Read the model definition and answer for the solid it produces. Units are mm, in the model's axes. A direction names the side the tool comes from. Round coordinates to 2 decimals unless told otherwise and drop trailing zeros. Write each loop counter-clockwise with the first axis right and the second up, starting at its lowest first coordinate (ties: lowest second). Pieces come first, ordered by that corner, then holes. Notation, with made-up numbers: (49, -23) -> (84, -23) arc R27 cw to (84, 0) -> close; hole circle Ø5 at (48, 16.5). An arc over 180 degrees is marked (long way). Return JSON: item names as keys, results as strings.
from build123d import *

# Parameters (mm, degrees)
F0_W     = 27
F0_H     = 19
F1_DEPTH = 2
F2_R     = 3.5
F3_R     = 0.5


with BuildPart() as f1:
    # F0 (on Front) → F1 (new body)
    with BuildSketch(Plane.XZ):
        with Locations((-46.395146, 6.552132)):
            Rectangle(F0_W, F0_H)
        with BuildLine():
            ThreePointArc((-45.395146, 12.252132), (-43.895146, 13.752132), (-42.395146, 12.252132))
            Line((-42.395146, 12.252132), (-42.395146, 8.716104))
            Line((-42.395146, 8.716104), (-39.834486, 6.155444))
            ThreePointArc((-39.834486, 6.155444), (-39.509326, 5.668809), (-39.395146, 5.094783))
            Line((-39.395146, 5.094783), (-39.395146, 2.152132))
            ThreePointArc((-39.395146, 2.152132), (-39.834486, 1.091472), (-40.895146, 0.652132))
            Line((-40.895146, 0.652132), (-43.895146, 0.652132))
            ThreePointArc((-43.895146, 0.652132), (-44.955806, 1.091472), (-45.395146, 2.152132))
            Line((-45.395146, 2.152132), (-45.395146, 2.652132))
            ThreePointArc((-45.395146, 2.652132), (-44.908531, 3.758048), (-43.764412, 4.146424))
            Line((-43.764412, 4.146424), (-41.90547, 3.983787))
            Line((-41.90547, 3.983787), (-41.955806, 4.034123))
            Line((-41.955806, 4.034123), (-45.395146, 7.473463))
            Line((-45.395146, 7.473463), (-45.395146, 12.252132))
        make_face(mode=Mode.SUBTRACT)
    extrude(amount=F1_DEPTH)

    # F2
    f2_edges = [f1.edges().sort_by_distance(p)[0] for p in [
        (-45.395146, -1, 7.473463),
    ]]
    fillet(f2_edges, radius=F2_R)

    # F3
    f3_edges = [f1.edges().sort_by_distance(p)[0] for p in [
        (-42.395146, -1, 8.716104),
    ]]
    fillet(f3_edges, radius=F3_R)


solid = f1.part
Item 1: Section B-B (y = -0.65) is taken. Give the vertices of the cut face in (x, z), then the cut area to 3 significant figures.
Worked answers:
{"outline": "(-59.9, -2.95) -> (-32.9, -2.95) -> (-32.9, 16.05) -> (-59.9, 16.05) -> close; hole (-45.4, 2.15) arc R1.5 ccw to (-43.9, 0.65) -> (-40.9, 0.65) arc R1.5 ccw to (-39.4, 2.15) -> (-39.4, 5.09) arc R1.5 ccw to (-39.83, 6.16) -> (-42.25, 8.57) arc R0.5 cw to (-42.4, 8.92) -> (-42.4, 12.25) arc R1.5 ccw to (-45.4, 12.25) -> (-45.4, 8.92) arc R3.5 ccw to (-44.37, 6.45) -> (-41.91, 3.98) -> (-43.76, 4.15) arc R1.5 ccw to (-45.4, 2.65) -> close", "area": "462 mm2"}
Item 2: A tool of negligible diameter and unlimited length cuts with its end or side. For faces 1 (the flat face through (-47, 0, 7)), 2 (the flat face through (-42, -1, 0.652)), from which of +Z, -Z, +X, -X, +Y, -Y can it reach the whole face along a straight path? Write none if from no direction.
Worked answers:
{"face 1": "+Z, -Z, +X, -X, +Y", "face 2": "+Y, -Y"}
Item 3: Section C-C (z = 5.5) is taken. Give the vertices of the cut face in (x, y).
Worked answers:
{"outline": "(-59.9, -2) -> (-43.42, -2) -> (-43.42, 0) -> (-59.9, 0) -> close; (-39.45, -2) -> (-32.9, -2) -> (-32.9, 0) -> (-39.45, 0) -> close"}
Item 4: Straight lines are drawn through the part: L1, parallel to X at y = -0.35, z = 9.5; L2, parallel to X at y = -1.85, z = 2.75; L3, parallel to Z at x = -44, y = -0.4. For each, find the intervals that lie inside material, in ascending order. Write a range as [from, to].
Worked answers:
{"L1": "x = [-59.9, -45.4], [-42.4, -32.9]", "L2": "x = [-59.9, -45.39], [-39.4, -32.9]", "L3": "z = [-2.95, 0.66], [4.15, 6.08], [13.75, 16.05]"}
Item 5: Section A-A (z = 10.5) is taken. Give the vertices of the cut face in (x, y), then the cut area to 3 significant figures.
Worked answers:
{"outline": "(-59.9, -2) -> (-45.4, -2) -> (-45.4, 0) -> (-59.9, 0) -> close; (-42.4, -2) -> (-32.9, -2) -> (-32.9, 0) -> (-42.4, 0) -> close", "area": "48.0 mm2"}
Item 6: For a pull along X with two mould halves and no side action, classify faces 3 (the flat face through (-59.895, -1, 6)), 4 (the flat face through (-47, -2, 7)), 5 (the flat face through (-43.12, -0.99, 5.2)) as released by +X, released by -X, zero draft, split by the parting line, or undercut.
Worked answers:
{"face 3": "released by -X", "face 4": "zero draft", "face 5": "undercut"}
